from build123d import *

# Parameters (mm, degrees)
BOSS_EXTRUDE1_DEPTH = 203.2
CUT_EXTRUDE1_DEPTH  = 12.7
CUT_EXTRUDE2_DEPTH  = 12.7
FILLET3_R           = 12.7


with BuildPart() as part:
    # Sketch1 → Boss-Extrude1 (new body)
    with BuildSketch(Plane.XY):
        Polygon((114.3, 41.748133631), (0, 41.748133631), (0, 29.141659697), (62.004048203, 29.141659697), (42.728136767, -11.95603827), (0, -11.95603827), (0, -24.500078422), (77.843883309, -24.500078422), align=None)
        Polygon((0, 41.748133631), (-114.3, 41.748133631), (-77.843883309, -24.500078422), (0, -24.500078422), (0, -11.95603827), (-42.728136767, -11.95603827), (-62.004048203, 29.141659697), (0, 29.141659697), align=None)
        Polygon((62.004048203, 29.141659697), (0, 29.141659697), (0, 0), (0, -11.95603827), (42.728136767, -11.95603827), align=None)
        Polygon((0, 0), (0, 29.141659697), (-62.004048203, 29.141659697), (-42.728136767, -11.95603827), (0, -11.95603827), align=None)
    extrude(amount=BOSS_EXTRUDE1_DEPTH)

    # Sketch2 → Cut-Extrude1 (cut)
    with BuildSketch(Plane(origin=(0, 0, 0), x_dir=(-1, 0, 0), z_dir=(0, 0, -1))):
        Polygon((61.610965664, 33.637347898), (-61.610965664, 33.637347898), (-40.398919629, -12.294528868), (40.398919629, -12.294528868), align=None)
    extrude(amount=-CUT_EXTRUDE1_DEPTH, mode=Mode.SUBTRACT)

    # Sketch3 → Cut-Extrude2 (cut)
    with BuildSketch(Plane.XY.offset(203.2)):
        Polygon((71.075916858, 34.413325386), (-71.075916858, 34.413325386), (-43.162708171, -15.225650552), (43.162708171, -15.225650552), align=None)
    extrude(amount=-CUT_EXTRUDE2_DEPTH, mode=Mode.SUBTRACT)

    # Fillet3
    fillet3_edges = [part.edges().sort_by_distance(p)[0] for p in [
        (77.843883309, -24.500078422, 101.6),
        (-77.843883309, -24.500078422, 101.6),
    ]]
    fillet(fillet3_edges, radius=FILLET3_R)


solid = part.part
Design review of the part built by this model. Coordinates are the model's own, in mm. A direction names the side the tool comes from. Coordinates: 2 decimals unless noted, no trailing zeros. Order: outer loops, then holes, each group sorted by start corner. A loop starts at its lowest first (then second) coordinate and runs counter-clockwise, first axis right, second up. Notation, with made-up numbers: (59.25, -10) - (68.25, -10) arc R17 cw to (68.25, -4) - close; hole circle Ø3 at (79, 64). An arc over 180 degrees is marked (long way). Put each result on its own line as item: value.
1) The part is to be moulded in two halves that separate along X. For faces 4 (the face through (97.65, 11.49, 100.18)), 5 (the face through (56.9, 9.2, 196.9)), 6 (the face through (-1, -24.5, 100)), 7 (the face through (-1, -15.226, 197)), say which applies: released by +X, released by -X, zero draft, split by the parting line, or undercut.
Response values:
face 4: released by +X
face 5: undercut
face 6: zero draft
face 7: undercut
2) Take a section at A-A, the plane x = -36.5. Give the boundary of the cut face in (y, z).
Response values:
outline: (-24.5, 0) - (-12.29, 0) - (-12.29, 12.7) - (33.64, 12.7) - (33.64, 0) - (41.75, 0) - (41.75, 203.2) - (34.41, 203.2) - (34.41, 190.5) - (-15.23, 190.5) - (-15.23, 203.2) - (-24.5, 203.2) - close
3) Insertion check: P1, Ø2, axis at x = -43.5, y = 0.5, coming from the -Z side; P2, Ø15, axis at x = -25.5, y = 19.5, coming from the +Z side; P3, Ø6, axis at y = -9, z = 72.5, coming from the +X side. Each pin has a flat end and moves straight along its axis. Give the tip position at first contact, or say it passes through.
Response values:
P1: stops at z = 12.7
P2: stops at z = 190.5
P3: stops at x = 88.02
4) Take a section at B-B, the plane z = 104.5. Give the boundary of the cut face in (x, y), and give its area (3 significant figures).
Response values:
outline: (-114.3, 41.75) - (-81.46, -17.92) arc R12.7 ccw to (-70.34, -24.5) - (70.34, -24.5) arc R12.7 ccw to (81.46, -17.92) - (114.3, 41.75) - close
area: 12,700 mm²
5) Wall thickness on L1, parallel to Z at x = -37, y = 30.5; L2, parallel to X at y = -18, z = 27; L3, parallel to Y at x = 100.5, z = 157: over which ranges is each line inside the solid? List them lowest first. Write a range as from..to.
Response values:
L1: z = 12.7..190.5
L2: x = -81.42..81.42
L3: y = 16.67..41.75
6) Take a section at D-D, the plane y = 37.5. Give the boundary of the cut face in (x, z), and give its area (3 significant figures).
Response values:
outline: (-111.96, 0) - (111.96, 0) - (111.96, 203.2) - (-111.96, 203.2) - close
area: 45,500 mm²
7) Take a section at C-C, the plane y = -8. Give the boundary of the cut face in (x, z).
Response values:
outline: (-86.92, 0) - (-42.38, 0) - (-42.38, 12.7) - (42.38, 12.7) - (42.38, 0) - (86.92, 0) - (86.92, 203.2) - (47.23, 203.2) - (47.23, 190.5) - (-47.23, 190.5) - (-47.23, 203.2) - (-86.92, 203.2) - close
8) Tool access review of faces 1 (the face through (-1, 33.637, 6)), 2 (the face through (-2, -13, 0)), 3 (the face through (-1, 10, 190.5)): name each direction out of +Z, -Z, +X, -X, +Y, -Y from which nothing blocks a thin tool from reaching the whole face with its end or side.
Response values:
face 1: -Z
face 2: -Z, +X, -X, +Y, -Y
face 3: +Z
